Study the drawing (mm; zero at the part's minimum x, y, z) and answer. Round coordinates to 2 decimals unless told otherwise and drop trailing zeros. Loops run counter-clockwise (first coordinate to the right, second up) from the corner with the lowest first, then second, coordinate; pieces in that order, holes last. Notation, with made-up numbers: (18.25, -6) - (29.25, -6) arc R12 ccw to (29.25, 2) - close; hole circle Ø10 at (72, -18.75). An arc over 180 degrees is marked (long way). One line per item, written item: value.
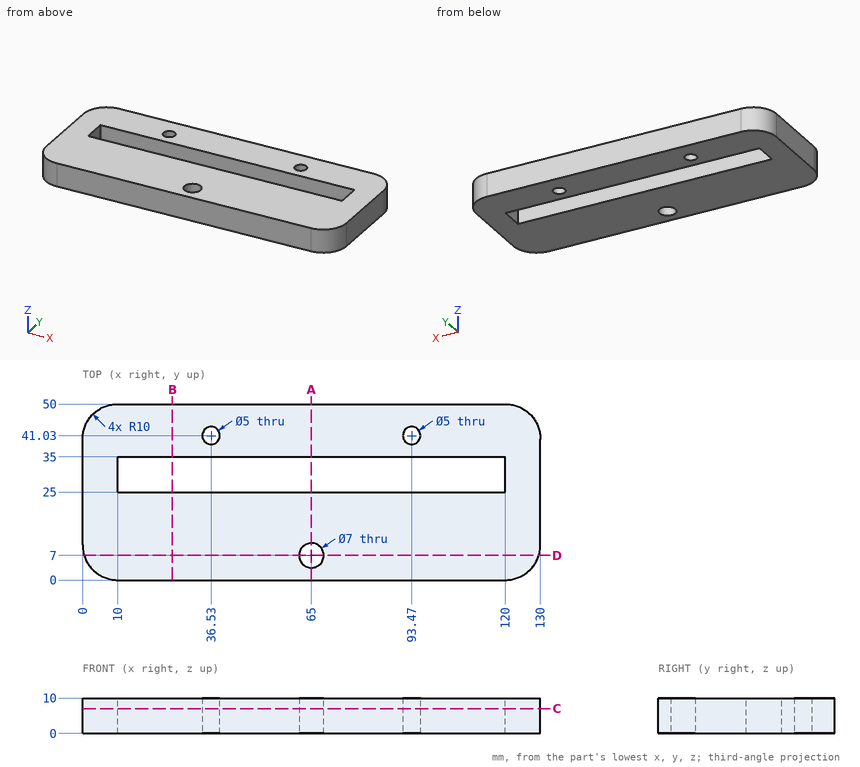
1) A cutting plane is placed at B-B on x = 25.5. Give the vertices of the cut face in (y, z).
Final values:
outline: (0, 0) - (25, 0) - (25, 10) - (0, 10) - close; (35, 0) - (50, 0) - (50, 10) - (35, 10) - close
2) A cutting plane is placed at A-A on x = 65. Give the vertices of the cut face in (y, z), and give its area (3 significant figures).
Final values:
outline: (0, 0) - (3.5, 0) - (3.5, 10) - (0, 10) - close; (10.5, 0) - (25, 0) - (25, 10) - (10.5, 10) - close; (35, 0) - (50, 0) - (50, 10) - (35, 10) - close
area: 330 mm2
3) Consider L1, parallel to Y at x = 36.53, z = 5; L2, parallel to Y at x = 65, z = 6; L3, parallel to Y at x = 45.5, z = 3.5. Determine where each line is inside the solid, lowest interval first.
Final values:
L1: 0 to 25, 35 to 38.53, 43.53 to 50
L2: 0 to 3.5, 10.5 to 25, 35 to 50
L3: 0 to 25, 35 to 50
4) A cutting plane is placed at D-D on y = 7. Give the vertices of the cut face in (x, z).
Final values:
outline: (0.46, 0) - (61.5, 0) - (61.5, 10) - (0.46, 10) - close; (68.5, 0) - (129.54, 0) - (129.54, 10) - (68.5, 10) - close
5) A cutting plane is placed at C-C on z = 7. Give the vertices of the cut face in (x, y).
Final values:
outline: (0, 10) arc R10 ccw to (10, 0) - (120, 0) arc R10 ccw to (130, 10) - (130, 40) arc R10 ccw to (120, 50) - (10, 50) arc R10 ccw to (0, 40) - close; hole (10, 25) - (120, 25) - (120, 35) - (10, 35) - close; hole circle Ø5 at (36.53, 41.03); hole circle Ø7 at (65, 7); hole circle Ø5 at (93.47, 41.03)
